Check sheet for the drawn part. Datum: minimum x, y, z corner. Units: mm. A direction names the side the tool comes from. Coordinates: 2 decimals unless noted, no trailing zeros. Loops run counter-clockwise (first coordinate to the right, second up) from the corner with the lowest first, then second, coordinate; pieces in that order, holes last.
Q1. Sectioned sample at A-A (x = 11). Enter the section's corners in (y, z), then the cut area to 3 significant figures.
Q2. Material ranges on probe 1 along Z at (x, y) = (7.75, 19.25); probe 2 along X at (y, z) = (12.5, 0.5); probe 3 along X at (y, z) = (17, 5.5), recorded low to high.
Q3. Go/stop test with flat-tipped pins: P1, Ø1, axis at x = 3.5, y = 4, coming from the -Z side; P2, Ø3.5, axis at y = 9, z = 1.5, coming from the +X side; P3, Ø3.5, axis at x = 9, z = 1, coming from the -Y side. Record where each tip stops, or that it passes through.
Q4. Access from +Z, -Z, +X, -X, +Y, -Y to the whole of each face (thin tool, end or side, straight path). Record for the marked faces 1, 2 and 3.
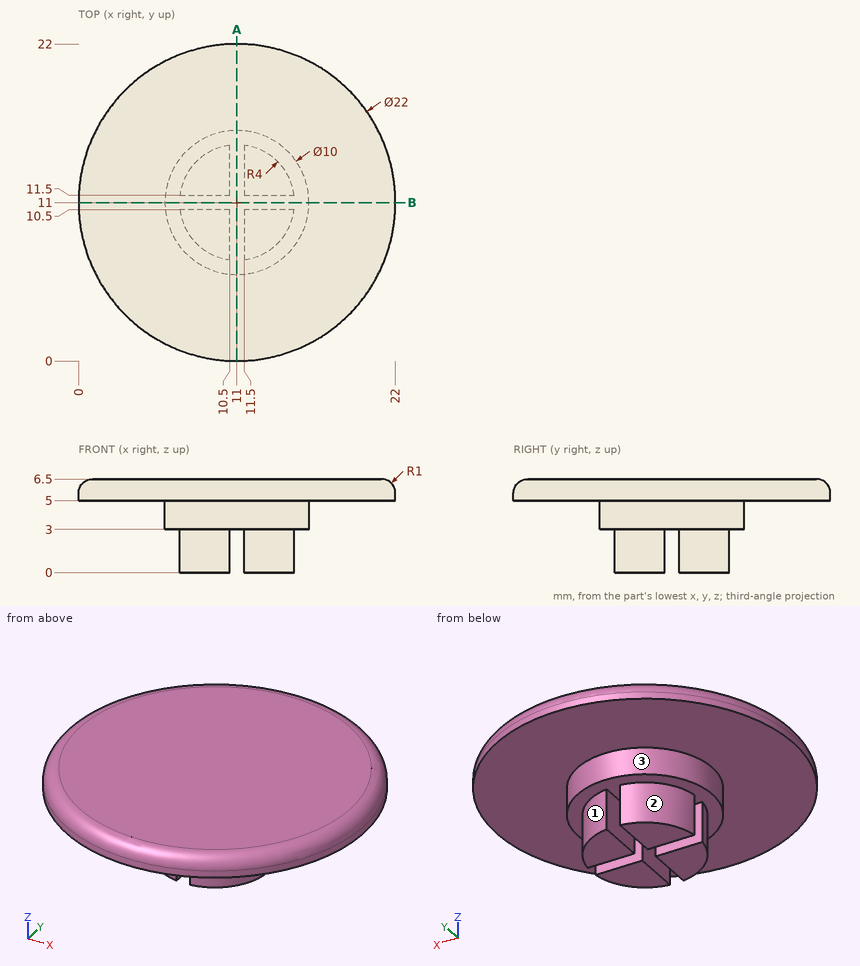
Geometry check:
1. outline: (0, 5) - (6, 5) - (6, 3) - (16, 3) - (16, 5) - (22, 5) - (22, 5.5) arc R1 ccw to (21, 6.5) - (1, 6.5) arc R1 ccw to (0, 5.5) - close
1. area: 52.6 mm2
2. probe 1: z = 5 to 6.5
2. probe 2: x = 7.29 to 10.5, 11.5 to 14.71
2. probe 3: x = 1.78 to 20.22
3. P1: stops at z = 5
3. P2: stops at x = 15.88
3. P3: stops at y = 7.03
4. face 1: -Z, +X, +Y
4. face 2: -Z, -X, +Y
4. face 3: -Z
